Can you work these out from the model? Positions are in its coordinate system, mm. Round coordinates to 2 decimals unless told otherwise and drop trailing zeros. Loops run counter-clockwise (first coordinate to the right, second up) from the corner with the lowest first, then second, coordinate; pieces in that order, holes last.
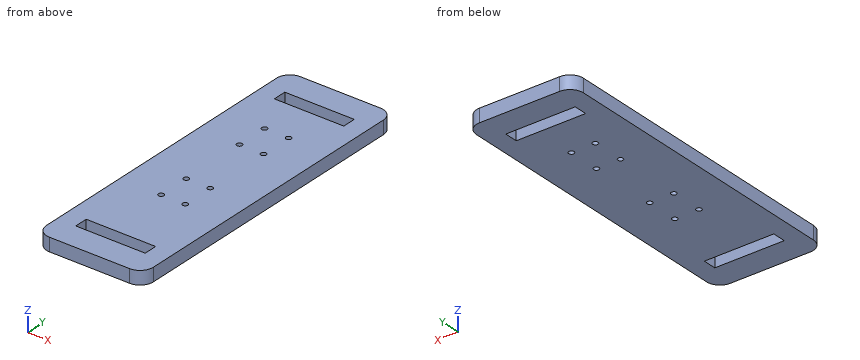
from build123d import *

# Parameters (mm, degrees)
SKETCH1_W           = 80
SKETCH1_H           = 240
BOSS_EXTRUDE1_DEPTH = 10
FILLET2_R           = 10
SKETCH2_R           = 2
SKETCH2_W           = 52
SKETCH2_H           = 10
CUT_EXTRUDE1_DEPTH  = 10


with BuildPart() as part:
    # Sketch1 → Boss-Extrude1 (new body)
    with BuildSketch(Plane.XY):
        with Locations((-40, 120)):
            Rectangle(SKETCH1_W, SKETCH1_H)
    extrude(amount=BOSS_EXTRUDE1_DEPTH)

    # Fillet2
    fillet2_edges = [part.edges().sort_by_distance(p)[0] for p in [
        (0, 0, 5),
        (-80, 0, 5),
        (-80, 240, 5),
        (0, 240, 5),
    ]]
    fillet(fillet2_edges, radius=FILLET2_R)

    # Sketch2 → Cut-Extrude1 (cut)
    with BuildSketch(Plane.XY.offset(10)):
        with Locations((-49, 154.94)):
            Circle(SKETCH2_R)
        with Locations((-31, 154.94)):
            Circle(SKETCH2_R)
        with Locations((-31, 178.94)):
            Circle(SKETCH2_R)
        with Locations((-49, 178.94)):
            Circle(SKETCH2_R)
        with Locations((-49, 103.94)):
            Circle(SKETCH2_R)
        with Locations((-49, 79.94)):
            Circle(SKETCH2_R)
        with Locations((-31, 103.94)):
            Circle(SKETCH2_R)
        with Locations((-31, 79.94)):
            Circle(SKETCH2_R)
        with Locations((-40, 215)):
            Rectangle(SKETCH2_W, SKETCH2_H)
        with Locations((-40, 25)):
            Rectangle(SKETCH2_W, SKETCH2_H)
    extrude(amount=-CUT_EXTRUDE1_DEPTH, mode=Mode.SUBTRACT)


solid = part.part
(1) If I drill on line 1 (Y direction, x = -57.5, z = 3); line 2 (X direction, y = 154.94, z = 2); line 3 (Y direction, x = -4.5, z = 7.5), over which ranges is the centre line in solid material (lowest first)?
Worked answers:
line 1: y = 0 to 20, 30 to 210, 220 to 240
line 2: x = -80 to -51, -47 to -33, -29 to 0
line 3: y = 1.65 to 238.35
(2) If we section it at A-A, the plane z = 3.75: State how many separate pieces and enclosed holes the cut face has, then the cut area to 3 significant figures.
Worked answers:
separate pieces: 1
enclosed holes: 10
area: 18,000 mm2
(3) If we section it at B-B, the plane x = -43.5: List the corners of the cut face in (y, z) for me.
Worked answers:
outline: (0, 0) - (20, 0) - (20, 10) - (0, 10) - close; (30, 0) - (210, 0) - (210, 10) - (30, 10) - close; (220, 0) - (240, 0) - (240, 10) - (220, 10) - close
